Work out the finished part from the listing and answer in its coordinate system (mm). Give positions to 0.01 mm unless a question says otherwise; leave off trailing zeros. Loops run counter-clockwise (first coordinate to the right, second up) from the corner with the lowest first, then second, coordinate; pieces in that order, holes last. Notation, with made-up numbers: M 24.5,11.25 L 47.5,11.25 A20 ccw 47.5,33.25 Z; hole C -24.5,-10.5 d3. An arc over 180 degrees is marked long. Write item = value, one per line. Start each with the question number.
1. Consider L1, parallel to Z at x = 3.75, y = -1; L2, parallel to Z at x = -3.5, y = -6; L3, parallel to X at y = -1.5, z = 1.75. Determine where each line is inside the solid, lowest interval first. Write a range as [from, to].
2. Section C-C on z = 2 is taken. Determine the outline of the cut face in (x, y).
3. Section B-B on z = 9.5 is taken. Determine the outline of the cut face in (x, y), plus the area to 3 significant figures.
4. Section A-A on z = 8 is taken. Determine the outline of the cut face in (x, y).
5. The mould has two halves that part along X. Classify faces 1 (the face through (0, 0, 15)), 2 (the face through (-0.501, 2.258, 5.313)), 3 (the face through (-0.62, 2.78, 2.85)): released by +X, released by -X, zero draft, split by the parting line, or undercut.
6. Flat-ended cylindrical pins translate along their axes: pin 1 Ø5 at (x, y) = (-7.5, -0.5) entering from +Z; pin 2 Ø10 at (x, y) = (-6.5, -3.5) entering from -Z; pin 3 Ø3 at (x, y) = (-2, -2.5) entering from -Z. Find the tip coordinate at first contact, or state that the pin passes through.
```python
from build123d import *

# Parameters (mm, degrees)
F4_R          = 2
F5_DEPTH      = 5
F5_DEPTH_BACK = 8


with BuildPart() as f1:
    # F0 (on Front) → F1 (revolve)
    with BuildSketch(Plane.XZ):
        Polygon((0, 10), (0, 0), (10, 10), align=None)
    revolve(axis=Axis((0, 0, 5), (0, 0, -1)))

    # F2 (on Front) → F3 (revolve, cut)
    with BuildSketch(Plane.XZ):
        Polygon((7, 10), (0, 10), (0, 3), align=None)
    revolve(axis=Axis((0, 0, 6.5), (0, 0, -1)), mode=Mode.SUBTRACT)

    # F4 (on face) → F5 (join, two sides)
    with BuildSketch(Plane.XY.offset(10)) as f5_sk:
        Circle(F4_R)
    extrude(amount=F5_DEPTH)
    extrude(f5_sk.sketch, amount=-F5_DEPTH_BACK)


solid = f1.part
```
Verdict:
q1.L1 = [3.88, 6.88]
q1.L2 = [6.95, 9.95]
q1.L3 = [-0.9, 0.9]
q2.outline = C 0,0 d4
q3.outline = C 0,0 d19; C 0,0 d4; hole C 0,0 d13
q3.area = 163 mm2
q4.outline = C 0,0 d16; C 0,0 d4; hole C 0,0 d10
q5.face_1 = zero draft
q5.face_2 = undercut
q5.face_3 = split by the parting line
q6.pin_1 = 10
q6.pin_2 = 2.38
q6.pin_3 = 1.7
